```python
from build123d import *

# Parameters (mm, degrees)
SKETCH1_W             = 8.88
SKETCH1_H             = 10
SKETCH1_R             = 1.6
BOSS_EXTRUDE1_DEPTH   = 1.4
BOSS_EXTRUDE1_2_DEPTH = 1.4
BOSS_EXTRUDE3_START   = -4
SKETCH1_5_W           = 34.26
SKETCH1_5_H           = 10
SKETCH1_5_R           = 1.6
BOSS_EXTRUDE3_DEPTH   = 4


with BuildPart() as part:
    # Sketch1 → Boss-Extrude1 (new body)
    with BuildSketch(Plane(origin=(0, 0, 0), x_dir=(1, 0, 0), z_dir=(0, 1, 0))):
        with Locations((4.44, 5)):
            Rectangle(SKETCH1_W, SKETCH1_H)
        with Locations(Location((4.44, 5, 0), (0, 0, 270))):
            Circle(SKETCH1_R, mode=Mode.SUBTRACT)
    extrude(amount=BOSS_EXTRUDE1_DEPTH)



with BuildPart() as body_2:
    # Sketch1 → Boss-Extrude1 2 (new body)
    with BuildSketch(Plane(origin=(0, 0, 0), x_dir=(1, 0, 0), z_dir=(0, 1, 0))):
        with Locations((29.82, 5)):
            Rectangle(SKETCH1_W, SKETCH1_H)
        with Locations(Location((29.82, 5, 0), (0, 0, 270))):
            Circle(SKETCH1_R, mode=Mode.SUBTRACT)
    extrude(amount=BOSS_EXTRUDE1_2_DEPTH)


with BuildPart() as part_1:
    add(part.part)

    add(body_2.part)  # Boss-Extrude3 merges body 2
    # Sketch1_5 → Boss-Extrude3 (add)
    with BuildSketch(Plane(origin=(0, 0, 0), x_dir=(1, 0, 0), z_dir=(0, 1, 0)).offset(BOSS_EXTRUDE3_START)):
        with Locations((17.13, 5)):
            Rectangle(SKETCH1_5_W, SKETCH1_5_H)
        with Locations(Location((4.44, 5, 0), (0, 0, 270))):
            Circle(SKETCH1_5_R, mode=Mode.SUBTRACT)
        with Locations(Location((29.82, 5, 0), (0, 0, 270))):
            Circle(SKETCH1_5_R, mode=Mode.SUBTRACT)
    extrude(amount=BOSS_EXTRUDE3_DEPTH)


solid = part_1.part
```
Work out the finished part from the listing and answer in its coordinate system (mm). A direction names the side the tool comes from. Give positions to 0.01 mm unless a question says otherwise; leave off trailing zeros. Write each loop counter-clockwise with the first axis right and the second up, starting at its lowest first coordinate (ties: lowest second). Pieces come first, ordered by that corner, then holes.
(1) The part is cut by section C-C on z = -5. Write down the section's boundary in (x, y).
Final values:
outline: (0, -4) - (2.84, -4) - (2.84, 1.4) - (0, 1.4) - close; (6.04, -4) - (28.22, -4) - (28.22, 1.4) - (25.38, 1.4) - (25.38, 0) - (8.88, 0) - (8.88, 1.4) - (6.04, 1.4) - close; (31.42, -4) - (34.26, -4) - (34.26, 1.4) - (31.42, 1.4) - close
(2) The part is cut by section D-D on y = -1.05. Write down the section's boundary in (x, z), plus the area to 3 significant figures.
Final values:
outline: (0, -10) - (34.26, -10) - (34.26, 0) - (0, 0) - close; hole circle Ø3.2 at (4.44, -5); hole circle Ø3.2 at (29.82, -5)
area: 327 mm2
(3) The part is cut by section B-B on x = 29.82. Write down the section's boundary in (y, z), plus the area to 3 significant figures.
Final values:
outline: (-4, -10) - (1.4, -10) - (1.4, -6.6) - (-4, -6.6) - close; (-4, -3.4) - (1.4, -3.4) - (1.4, 0) - (-4, 0) - close
area: 36.7 mm2
(4) Straight lines are drawn through the part: line 1 (X direction, y = -0.85, z = -5); line 2 (X direction, y = 0.3, z = -5); line 3 (X direction, y = 0.95, z = -3.75). For each, find the intervals that lie inside material, in ascending order.
Final values:
line 1: x = 0 to 2.84, 6.04 to 28.22, 31.42 to 34.26
line 2: x = 0 to 2.84, 6.04 to 8.88, 25.38 to 28.22, 31.42 to 34.26
line 3: x = 0 to 3.44, 5.44 to 8.88, 25.38 to 28.82, 30.82 to 34.26
(5) The part is cut by section A-A on y = 0.35. Write down the section's boundary in (x, z), plus the area to 3 significant figures.
Final values:
outline: (0, -10) - (8.88, -10) - (8.88, 0) - (0, 0) - close; (25.38, -10) - (34.26, -10) - (34.26, 0) - (25.38, 0) - close; hole circle Ø3.2 at (4.44, -5); hole circle Ø3.2 at (29.82, -5)
area: 162 mm2
(6) The mould has two halves that part along X. Classify faces 1 (the flat face through (0, -1, -5)), 2 (the flat face through (34.26, -1, -5)), 3 (the flat face through (2, 1.4, -5)), 4 (the cylindrical face through (6.026, -1.338, -5.208)): pulls with the +X half, pulls with the -X half, needs draft (parallel to the pull), parting line crosses it, or undercut.
Final values:
face 1: pulls with the -X half
face 2: pulls with the +X half
face 3: needs draft
face 4: undercut
(7) A flat-ended cylindrical pin translates along its axis: pin 1 Ø5 at (x, z) = (19.5, -7) entering from +Y. Find the tip coordinate at first contact, or state that the pin passes through.
Final values:
pin 1: stops at y = 0
(8) Which of the six approach directions +Z, -Z, +X, -X, +Y, -Y give full straight-line access (tool end or side, diameter ignored) to faces 5 (the flat face through (17, -1, 0)), 6 (the flat face through (25.38, 1, -5))?
Final values:
face 5: +Z, +X, -X, +Y, -Y
face 6: +Z, -Z, +Y
